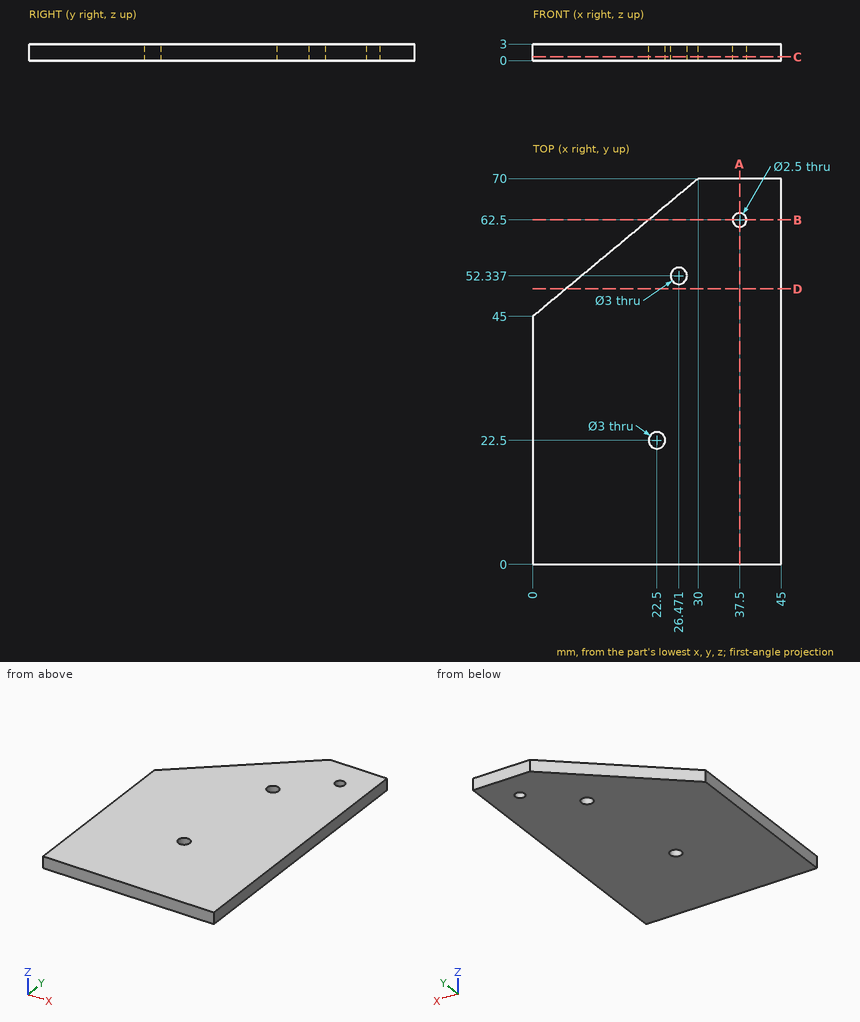
Drawing for the job (mm, zero at the part's lowest x, y, z). Round coordinates to 2 decimals unless told otherwise and drop trailing zeros. Loops run counter-clockwise (first coordinate to the right, second up) from the corner with the lowest first, then second, coordinate; pieces in that order, holes last. Notation, with made-up numbers: (24.25, 5) - (60.25, 5) arc R16 ccw to (60.25, 27) - close; hole circle Ø3 at (52, 62). An arc over 180 degrees is marked (long way). Return JSON: item names as keys, results as strings. Group by question number.
Q1. Band-saw the part on C-C on z = 0.65. Give the cut face in (x, y).
Q2. Band-saw the part on B-B on y = 62.5. Give the cut face in (x, z).
Q3. Flat gauge pins, fed straight in: pin 1 Ø2.5 at (x, y) = (22.5, 22.5) entering from +Z; pin 2 Ø1 at (x, z) = (18.5, 0.5) entering from +Y. Where does each tip first touch, or does it go through?
Q4. Drill centre lines: line 1 along X through (y, z) = (22.5, 0.8); line 2 along X through (y, z) = (62.5, 1.85); line 3 along Y through (x, z) = (22.5, 1.5). Where is each one in solid material? Low to high. Write a range as [from, to].
Q5. Band-saw the part on D-D on y = 50. Give the cut face in (x, z).
Q6. Band-saw the part on A-A on x = 37.5. Give the cut face in (y, z).
Solutions:
{
 "1": {"outline": "(0, 0) - (45, 0) - (45, 70) - (30, 70) - (0, 45) - close; hole circle Ø3 at (22.5, 22.5); hole circle Ø3 at (26.47, 52.34); hole circle Ø2.5 at (37.5, 62.5)"},
 "2": {"outline": "(21, 0) - (36.25, 0) - (36.25, 3) - (21, 3) - close; (38.75, 0) - (45, 0) - (45, 3) - (38.75, 3) - close"},
 "3": {"pin 1": "passes through", "pin 2": "stops at y = 60.83"},
 "4": {"line 1": "x = [0, 21], [24, 45]", "line 2": "x = [21, 36.25], [38.75, 45]", "line 3": "y = [0, 21], [24, 63.75]"},
 "5": {"outline": "(6, 0) - (45, 0) - (45, 3) - (6, 3) - close"},
 "6": {"outline": "(0, 0) - (61.25, 0) - (61.25, 3) - (0, 3) - close; (63.75, 0) - (70, 0) - (70, 3) - (63.75, 3) - close"}
}
